```python
from build123d import *

# Parameters (mm, degrees)
SKETCH_W     = 700
SKETCH_H     = 500
PAD_DEPTH    = 350
SKETCH001_R  = 40
PAD001_DEPTH = 30
SKETCH002_R  = 100
PAD002_DEPTH = 50


with BuildPart() as part:
    # Sketch → Pad (new body)
    with BuildSketch(Plane.XY):
        Rectangle(SKETCH_W, SKETCH_H)
    extrude(amount=PAD_DEPTH)

    # Sketch001 (on Face6 of Pad) → Pad001 (join)
    with BuildSketch(Plane.XY.offset(350)):
        Circle(SKETCH001_R)
    extrude(amount=PAD001_DEPTH)

    # Sketch002 (on Face6 of Pad001) → Pad002 (join)
    with BuildSketch(Plane.XZ.offset(250)):
        with Locations((-230, 0)):
            Circle(SKETCH002_R)
    pad002 = extrude(amount=PAD002_DEPTH)

    # Mirrored: Pad002 across XZ
    add(pad002.mirror(Plane.XZ))


solid = part.part
```
CAD build for the part. Positions are in the model's coordinates, mm. A direction names the side the tool comes from. Round coordinates to 2 decimals unless told otherwise and drop trailing zeros. Order: outer loops, then holes, each group sorted by start corner. A loop starts at its lowest first (then second) coordinate and runs counter-clockwise, first axis right, second up.
Item 1: Mould opens along Y. For faces 1 (the face through (-329.903, -274.65, 4.397)), 2 (the face through (-5, 250, 173)), 3 (the face through (-5, 4, 0)), 4 (the face through (-231, -250, -38)) say: pulls with the +Y half, pulls with the -Y half, needs draft (parallel to the pull), parting line crosses it, or undercut.
Item 2: Saw through at D-D on x = 0. Write the cut outline in (y, z).
Item 3: Saw through at B-B on y = 0. Write the cut outline in (x, z).
Item 4: Saw through at C-C on z = 109. Write the cut outline in (x, y).
Item 5: Tool access for faces 5 (the face through (-329.903, 274.65, 4.397)), 6 (the face through (-8.67, -39.05, 364.79)), 7 (the face through (-231, 250, -38)): list every direction of +Z, -Z, +X, -X, +Y, -Y with a clear straight run to the whole face (end or side of a thin tool).
Item 6: Saw through at A-A on x = -230. Write the cut outline in (y, z), then the cut area to 3 significant figures.
Item 7: Probe line 1 along Y through (x, z) = (272, 227.5); line 2 along Z through (x, y) = (260.5, 234); line 3 along Y through (x, z) = (-207, -46.5). List the from-to ranges inside material, lowest first.
Item 8: Pin check, flat tips, straight feed: pin 1 (2 mm diameter, centred on x = -156.5, y = 121.5, fed in from -Z); pin 2 (1 mm diameter, centred on x = -197, y = -231, fed in from +Z); pin 3 (1 mm diameter, centred on x = -116.5, z = 211, fed in from -Y). Stop position of each tip, or through.
Reported:
1. face 1: needs draft
1. face 2: pulls with the +Y half
1. face 3: undercut
1. face 4: undercut
2. outline: (-250, 0) - (250, 0) - (250, 350) - (40, 350) - (40, 380) - (-40, 380) - (-40, 350) - (-250, 350) - close
3. outline: (-350, 0) - (350, 0) - (350, 350) - (40, 350) - (40, 380) - (-40, 380) - (-40, 350) - (-350, 350) - close
4. outline: (-350, -250) - (350, -250) - (350, 250) - (-350, 250) - close
5. face 5: +Y
5. face 6: +Z
5. face 7: -Z, +X, -X
6. outline: (-300, -100) - (-250, -100) - (-250, 0) - (250, 0) - (250, -100) - (300, -100) - (300, 100) - (250, 100) - (250, 350) - (-250, 350) - (-250, 100) - (-300, 100) - close
6. area: 195,000 mm2
7. line 1: y = -250 to 250
7. line 2: z = 0 to 350
7. line 3: y = -300 to -250, 250 to 300
8. pin 1: stops at z = 0
8. pin 2: stops at z = 350
8. pin 3: stops at y = -250
